Geometry check sheet. Reference: the model listing, model coordinates, mm. A direction names the side the tool comes from. Round coordinates to 2 decimals unless told otherwise and drop trailing zeros. Order: outer loops, then holes, each group sorted by start corner. A loop starts at its lowest first (then second) coordinate and runs counter-clockwise, first axis right, second up.
(1) Thickness scan on L1, parallel to X at y = -27, z = 5.75; L2, parallel to Y at x = 28, z = 5.5; L3, parallel to X at y = -88, z = 2.75. Record the ranges inside material, lowest first.
(2) Cross-section at B-B on z = 5.5. Enter the section's corners in (x, y).
(3) Set-up check for faces 1 (the face through (9, 4, 7)), 2 (the face through (42, -16, 7)), 3 (the face through (45, -1, 7)), 4 (the face through (33, 10, 7)), 5 (the face through (-30.275, -91.161, 6.916)): record each of +Z, -Z, +X, -X, +Y, -Y from which the full face is reachable in a straight line by a thin tool's end or side.
(4) Cross-section at C-C on x = 3. Enter the section's corners in (y, z).
(5) Cross-section at A-A on y = 5.5. Enter the section's corners in (x, z), and give its area (3 significant figures).
(6) Gauge pin test, flat ends, axial feed: P1, Ø1, axis at y = -82, z = 8.5, coming from the +X side; P2, Ø5, axis at x = -13.5, z = 1.5, coming from the +Y side; P3, Ø6, axis at y = 0, z = 12, coming from the -X side. Record the tip position at first contact, or that the pin passes through.
(7) Cross-section at D-D on y = -32.5. Enter the section's corners in (x, z).
from build123d import *

# Parameters (mm, degrees)
F1_DEPTH = 14
F2_R     = 1


with BuildPart() as f1:
    # F0 (on Top) → F1 (new body)
    with BuildSketch(Plane.XY):
        with BuildLine():
            ThreePointArc((43.5, -16), (44.56066, -15.56066), (45, -14.5))
            Line((45, -14.5), (45, 12.5))
            ThreePointArc((45, 12.5), (44.56066, 13.56066), (43.5, 14))
            Line((43.5, 14), (22.5, 14))
            ThreePointArc((22.5, 14), (21.43934, 13.56066), (21, 12.5))
            Line((21, 12.5), (21, 4))
            Line((21, 4), (-3.5, 4))
            ThreePointArc((-3.5, 4), (-4.56066, 3.56066), (-5, 2.5))
            Line((-5, 2.5), (-5, -92.320508))
            ThreePointArc((-5, -92.320508), (-10, -100.980762), (-20, -100.980762))
            ThreePointArc((-20, -100.980762), (-30.384159, -90.988886), (-34.911111, -77.307692))
            ThreePointArc((-34.911111, -77.307692), (-35.705288, -75.665502), (-37.403703, -75))
            ThreePointArc((-37.403703, -75), (-39.238202, -75.801584), (-39.896296, -77.692308))
            ThreePointArc((-39.896296, -77.692308), (-28.777818, -100.682978), (-5, -110))
            ThreePointArc((-5, -110), (-1.464466, -108.535534), (0, -105))
            Line((0, -105), (0, 0))
            Line((0, 0), (23.5, 0))
            ThreePointArc((23.5, 0), (24.56066, 0.43934), (25, 1.5))
            Line((25, 1.5), (25, 10))
            Line((25, 10), (41, 10))
            Line((41, 10), (41, -16))
            Line((41, -16), (43.5, -16))
        make_face()
    extrude(amount=F1_DEPTH)

    # F2
    f2_edges = [f1.edges().sort_by_distance(p)[0] for p in [
        (45, -1, 14),
        (44.56066, 13.56066, 14),
        (33, 14, 14),
        (8.75, 4, 14),
        (-5, -44.910254, 0),
        (21, 8.25, 0),
    ]]
    fillet(f2_edges, radius=F2_R)


solid = f1.part
Found:
1. L1: x = -5 to 0
1. L2: y = 10 to 14
1. L3: x = -37.5 to -32.04, -5 to 0
2. outline: (-39.9, -77.69) arc R35 ccw to (-5, -110) arc R5 ccw to (0, -105) - (0, 0) - (23.5, 0) arc R1.5 ccw to (25, 1.5) - (25, 10) - (41, 10) - (41, -16) - (43.5, -16) arc R1.5 ccw to (45, -14.5) - (45, 12.5) arc R1.5 ccw to (43.5, 14) - (22.5, 14) arc R1.5 ccw to (21, 12.5) - (21, 4) - (-3.5, 4) arc R1.5 ccw to (-5, 2.5) - (-5, -92.32) arc R10 cw to (-20, -100.98) arc R30 cw to (-34.91, -77.31) arc R2.5 ccw to (-37.4, -75) arc R2.5 ccw to start
3. face 1: +Z, -Z, -X, +Y
3. face 2: +Z, -Z, +X, -Y
3. face 3: +Z, -Z, +X, +Y, -Y
3. face 4: +Z, -Z, -Y
3. face 5: +Z, -Z, +Y
4. outline: (0, 0) - (3, 0) arc R1 ccw to (4, 1) - (4, 13) arc R1 ccw to (3, 14) - (0, 14) - close
5. outline: (21, 1) arc R1 ccw to (22, 0) - (25, 0) - (25, 14) - (22, 14) arc R1 ccw to (21, 13) - close; (41, 0) - (44, 0) arc R1 ccw to (45, 1) - (45, 13) arc R1 ccw to (44, 14) - (41, 14) - close
5. area: 111 mm2
6. P1: stops at x = 0
6. P2: stops at y = -101.49
6. P3: stops at x = -5
7. outline: (-5, 1) arc R1 ccw to (-4, 0) - (-1, 0) arc R1 ccw to (0, 1) - (0, 13) arc R1 ccw to (-1, 14) - (-4, 14) arc R1 ccw to (-5, 13) - close
